For this review, take the finished solid that the model builds, in its own axes (mm). A direction names the side the tool comes from. Round coordinates to 2 decimals unless told otherwise and drop trailing zeros. Write each loop counter-clockwise with the first axis right and the second up, starting at its lowest first coordinate (ties: lowest second). Pieces come first, ordered by that corner, then holes. Notation, with made-up numbers: (-24.5, 77.25) -> (11.5, 77.25) arc R20 cw to (11.5, 107.25) -> close; hole circle Ø9 at (-29, 76). An arc over 180 degrees is marked (long way). Answer as CSV lines item,"result". Start each with the question number.
Item 1: Take a section at A-A on z = 100. Give the boundary of the cut face in (x, y), then the cut area to 3 significant figures.
Item 2: Wall thickness on probe 1 along X at (y, z) = (-55, 110); probe 2 along Z at (x, y) = (-14, -19); probe 3 along X at (y, z) = (-91.5, 32): over which ranges is each line inside the solid? List them lowest first. Write a range as from..to.
Item 3: Machinability: for faces 1 (the flat face through (-18, -100, 56)), 2 (the flat face through (-30, -49, 84)), which of the approach directions +Z, -Z, +X, -X, +Y, -Y give a long, thin tool a straight path to every point of the face, cutting with its end or side? Answer none if there is none.
Item 4: For pin 1 Ø6 at (y, z) = (-50, 112.5) entering from -X; pin 2 Ø3 at (x, y) = (-52, -64) entering from +Z, all flat-tipped, find the tip position at first contact; note any pin that passes through.
```python
from build123d import *

# Parameters (mm, degrees)
F0_W     = 30
F0_H     = 110
F1_DEPTH = 100
F2_R     = 14.99999
F3_R     = 14.99999
F4_R     = 1.5


# Not quite as in the source:
# - a fillet or chamfer is up to 0.001 mm smaller than in the source, because OpenCascade refuses the exact size


with BuildPart() as f1:
    # F0 (on Front) → F1 (new body)
    with BuildSketch(Plane.XZ):
        Polygon((-60, 0), (0, 0), (0, 30), (-30, 30), (-60, 30), align=None)
        with Locations((-15, 85)):
            Rectangle(F0_W, F0_H)
    extrude(amount=F1_DEPTH)

    # F2 (radius 15 in the source; OpenCascade refuses exactly that, so slightly less here)
    f2_edges = [f1.edges().sort_by_distance(p)[0] for p in [
        (-30, -50, 30),
        (-60, -50, 30),
    ]]
    fillet(f2_edges, radius=F2_R)

    # F3 (radius 15 in the source; OpenCascade refuses exactly that, so slightly less here)
    f3_edges = [f1.edges().sort_by_distance(p)[0] for p in [
        (-30, -50, 140),
        (0, -50, 140),
    ]]
    fillet(f3_edges, radius=F3_R)

    # F4
    f4_edges = [f1.edges().sort_by_distance(p)[0] for p in [
        (0, -50, 0),
        (-30, -100, 0),
        (-60, -50, 0),
        (-30, 0, 0),
        (0, -100, 62.500005),
        (0, 0, 62.500005),
    ]]
    fillet(f4_edges, radius=F4_R)


solid = f1.part
```
Output values:
1,outline,"(-30, -98.5) arc R1.5 ccw to (-28.5, -100) -> (-1.5, -100) arc R1.5 ccw to (0, -98.5) -> (0, -1.5) arc R1.5 ccw to (-1.5, 0) -> (-28.5, 0) arc R1.5 ccw to (-30, -1.5) -> close"
1,area,"3,000 mm^2"
2,probe 1,"x = -30..0"
2,probe 2,"z = 0..139.97"
2,probe 3,"x = -37.52..0"
3,face 1,"+Z, -Z, +X, -X, -Y"
3,face 2,"+Z, -X, +Y, -Y"
4,pin 1,"stops at x = -30"
4,pin 2,"stops at z = 28.96"
